Autodesk Inventor part; units mm, degrees
ref_plane "YZ Plane" through (0, 0, 0) normal (1, 0, 0) x (0, 1, 0)
ref_plane "XZ Plane" through (0, 0, 0) normal (0, 1, 0) x (-1, 0, 0)
ref_plane "XY Plane" through (0, 0, 0) normal (0, 0, 1) x (1, 0, 0)
sketch "Sketch1" plane through (0, 0, 0) normal (0, 0, 1) x (1, 0, 0)
  line L0 (0, 0) -> (48, 0) construction
  line L1 (0, 46) -> (0, 66)
  line L2 (0, 66) -> (3, 66)
  line L3 (3, 107.5) -> (31, 107.5)
  line L4 (0, 46) -> (0, 0) construction
  line L5 (3, 107.5) -> (3, 66)
  line L6 (31, 107.5) -> (31, 61)
  line L7 (0, 46) -> (48, 46)
  line L8 (48, 46) -> (48, 0) construction
  line L9 (48, 59.5127) -> (31, 61)
  line L10 (48, 59.5127) -> (48, 46)
  dimension "d0" = 132
  dimension "d1" = 215
  dimension "d2" = 31
  dimension "d3" = 3
  dimension "d8" = 92
  dimension "d9" = 122
  dimension "d10" = 48
  dimension "d12" = 5
revolve "Revolution1" add sketch "Sketch1" angle 360 about axis through (0, 0, 0) along (1, 0, 0)
sketch "Sketch2" plane through (3, 0, 0) normal (-1, 0, 0) x (0, 0, 1)
  circle A0 centre (0, 0) radius 66
  line L0 (0, 0) -> (0, 85) construction
  circle A1 centre (0, 0) radius 107.5
  circle A2 centre (0, 0) radius 85 construction
  line L1 (0, 0) -> (32.5281, 78.5298) construction
  circle A3 centre (32.5281, 78.5298) radius 11.5
  dimension "d13" = 23
  dimension "d14" = 85
  dimension "d15" = 22.5
extrude "Extrusion1" cut sketch "Sketch2" against normal blind 31 contours A3
pattern_circular "Circular Pattern1" count 8 over 360 about axis through (1.5, 0, 0) along (1, 0, 0) of "Extrusion1"
equation "\"d0\" = D1"
equation "\"d1\" = D"
equation "\"d2\" = C1"
equation "\"d3\" = F1"
equation "\"d8\" = ID + 2 * t"
equation "\"d9\" = N3"
equation "\"d10\" = H2"
equation "\"d13\" = L"
equation "\"d14\" = 0.5 * K1"
equation "\"d4\" = C1"
equation "\"C1\" = 31"
equation "\"D\" = 215"
equation "\"L\" = 23"
equation "\"N3\" = 122"
equation "\"D1\" = 132"
equation "\"H2\" = 48"
equation "\"F1\" = 3"
equation "\"t\" = 6"
equation "\"Size_Designation\" = 1.2345"
properties part number "DIN EN 1092-2 Hubbed Slip-On Flange for Welding Type 12 - PN 63 Ductile Iron DN80" material "Iron, Ductile"
Can you work these out from the model? Positions are in its coordinate system, mm. A direction names the side the tool comes from. Round coordinates to 2 decimals unless told otherwise and drop trailing zeros. Write each loop counter-clockwise with the first axis right and the second up, starting at its lowest first coordinate (ties: lowest second). Pieces come first, ordered by that corner, then holes. Notation, with made-up numbers: (45.25, -12.5) - (92.25, -12.5) arc R12 cw to (92.25, 3.5) - close; hole circle Ø9 at (-6.75, 17.25). An arc over 180 degrees is marked (long way). Write each question's results on one line, items separated by ' | '. Start each with the question number.
1) Suppose I cut it at A-A (y = 0). List the corners of the cut face in (x, z) for me.
2) Suppose I cut it at D-D (x = 19). Give the number of separate pieces and of enclosed holes in the cut face, and give its area (3 significant figures).
3) We'd pull the mould along Y, two halves only. Please class faces 3 (the flat face through (3, -2, -70)), 4 (the cylindrical face through (1.521, 60.967, -25.278)), 5 (the cylindrical face through (16.804, 67.303, 30.035)): released by +Y, released by -Y, zero draft, split by the parting line, or undercut.
4) Which directions (+Z, -Z, +X, -X, +Y, -Y) give clear straight access to the entire face, cutting with the end or side of a thin tool? Please do faces 1 (the flat face through (31, 46, -46)), 2 (the cylindrical face through (16.804, -67.303, -30.035)).
5) For pin 1 Ø5 at (y, z) = (-55.5, -82.5) entering from +X; pin 2 Ø4 at (x, z) = (6, 21.5) entering from -Y; pin 3 Ø1 at (x, y) = (9, 18.5) entering from +Z, each with a flat end and sliding along its axis, tell me the tip position at first contact or that it passes through.
6) Suppose I cut it at C-C (y = 75.5). List the corners of the cut face in (x, z) for me.
7) Please list where these lines run through material, in increasing order: line 1 (Z direction, x = 28.5, y = 0); line 2 (Y direction, x = 26.5, z = 71); line 3 (Z direction, x = 10, y = -41.5).
Here are the results:
1) outline: (0, -66) - (3, -66) - (3, -107.5) - (31, -107.5) - (31, -61) - (48, -59.51) - (48, -46) - (0, -46) - close; (0, 46) - (48, 46) - (48, 59.51) - (31, 61) - (31, 107.5) - (3, 107.5) - (3, 66) - (0, 66) - close
2) separate pieces: 1 | enclosed holes: 9 | area: 26,300 mm2
3) face 3: zero draft | face 4: split by the parting line | face 5: undercut
4) face 1: +X | face 2: +X, -X
5) pin 1: stops at x = 31 | pin 2: stops at y = -105.72 | pin 3: stops at z = 105.98
6) outline: (3, -76.52) - (31, -76.52) - (31, -43.62) - (3, -43.62) - close; (3, -21.43) - (31, -21.43) - (31, 21.43) - (3, 21.43) - close; (3, 43.62) - (31, 43.62) - (31, 76.52) - (3, 76.52) - close
7) line 1: z = -107.5 to -46, 46 to 107.5 | line 2: y = -80.72 to -41.22, -23.84 to 23.84, 41.22 to 80.72 | line 3: z = -99.17 to -85.72, -71.34 to -19.84, 19.84 to 71.34, 85.72 to 99.17
